```python
from build123d import *

# Parameters (mm, degrees)
SKETCH2_W                    = 600
SKETCH2_H                    = 812
BASE_FLANGE1_DEPTH           = 2
EDGE_FLANGE1_STRIP_W         = 9
EDGE_FLANGE1_STRIP_H         = 2
EDGE_FLANGE1_STRIP_CUT_DEPTH = 600
EDGE_FLANGE1_DEPTH           = 600
EDGE_FLANGE3_DEPTH           = 809.5
EDGE_FLANGE4_DEPTH           = 809.5
EDGE_FLANGE5_DEPTH           = 600
SKETCH22_R                   = 2.5
CUT_EXTRUDE1_DEPTH           = 870.278724001
SKETCH23_R                   = 2.5
CUT_EXTRUDE2_DEPTH           = 870.278724001
SKETCH24_R                   = 2.5
CUT_EXTRUDE3_DEPTH           = 25
EDGE_FLANGE6_STRIP_W         = 10
EDGE_FLANGE6_STRIP_H         = 2
EDGE_FLANGE6_STRIP_CUT_DEPTH = 809.5
EDGE_FLANGE6_DEPTH           = 809.5
EDGE_FLANGE7_STRIP_W         = 10
EDGE_FLANGE7_STRIP_H         = 2
EDGE_FLANGE7_STRIP_CUT_DEPTH = 809.5
EDGE_FLANGE7_DEPTH           = 809.5
EDGE_FLANGE8_STRIP_W         = 10
EDGE_FLANGE8_STRIP_H         = 2
EDGE_FLANGE8_STRIP_CUT_DEPTH = 809.5
EDGE_FLANGE8_DEPTH           = 809.5
EDGE_FLANGE9_STRIP_W         = 10
EDGE_FLANGE9_STRIP_H         = 2
EDGE_FLANGE9_STRIP_CUT_DEPTH = 809.5
EDGE_FLANGE9_DEPTH           = 809.5


# Sheet-metal steps are written as plain solids
with BuildPart() as part:
    # Sketch2 → Base-Flange1 (new body)
    with BuildSketch(Plane(origin=(0, 0, 0), x_dir=(0, 0, -1), z_dir=(1, 0, 0))):
        Rectangle(SKETCH2_W, SKETCH2_H)
    extrude(amount=-BASE_FLANGE1_DEPTH)

    # Edge-Flange1 strip (across the edge) → Edge-Flange1 strip cut (cut)
    with BuildSketch(Plane(origin=(-2, 406, 300), x_dir=(0, -1, 0), z_dir=(0, 0, -1))):
        with Locations((-2, -1)):
            Rectangle(EDGE_FLANGE1_STRIP_W, EDGE_FLANGE1_STRIP_H)
    extrude(amount=EDGE_FLANGE1_STRIP_CUT_DEPTH, mode=Mode.SUBTRACT)

    # Edge-Flange1 section (across the edge) → Edge-Flange1 (add)
    with BuildSketch(Plane(origin=(-2, 406, 300), x_dir=(0, -1, 0), z_dir=(0, 0, -1))):
        with BuildLine():
            Line((0, 0.5), (0, 25))
            Line((0, 25), (2, 25))
            Line((2, 25), (2, 0.5))
            ThreePointArc((2, 0.5), (2.146446609, 0.146446609), (2.5, 0))
            Line((2.5, 0), (2.5, -2))
            ThreePointArc((2.5, -2), (0.732233047, -1.267766953), (0, 0.5))
        make_face()
    extrude(amount=EDGE_FLANGE1_DEPTH)

    # Edge-Flange3 section (across the edge) → Edge-Flange3 (add)
    with BuildSketch(Plane(origin=(-2, -406, 300.5), x_dir=(0, 0, -1), z_dir=(0, 1, 0))):
        with BuildLine():
            Line((-2, 0.5), (-2, 25))
            Line((-2, 25), (0, 25))
            Line((0, 25), (0, 0.5))
            ThreePointArc((0, 0.5), (0.146446609, 0.146446609), (0.5, 0))
            Line((0.5, 0), (0.5, -2))
            ThreePointArc((0.5, -2), (-1.267766953, -1.267766953), (-2, 0.5))
        make_face()
    extrude(amount=EDGE_FLANGE3_DEPTH)

    # Edge-Flange4 section (across the edge) → Edge-Flange4 (add)
    with BuildSketch(Plane(origin=(-2, 403.5, -300.5), x_dir=(0, 0, 1), z_dir=(0, -1, 0))):
        with BuildLine():
            Line((-2, 0.5), (-2, 25))
            Line((-2, 25), (0, 25))
            Line((0, 25), (0, 0.5))
            ThreePointArc((0, 0.5), (0.146446609, 0.146446609), (0.5, 0))
            Line((0.5, 0), (0.5, -2))
            ThreePointArc((0.5, -2), (-1.267766953, -1.267766953), (-2, 0.5))
        make_face()
    extrude(amount=EDGE_FLANGE4_DEPTH)

    # Edge-Flange5 section (across the edge) → Edge-Flange5 (add)
    with BuildSketch(Plane(origin=(-2, -406.5, -300), x_dir=(0, 1, 0), z_dir=(0, 0, 1))):
        with BuildLine():
            Line((-2, 0.5), (-2, 25))
            Line((-2, 25), (0, 25))
            Line((0, 25), (0, 0.5))
            ThreePointArc((0, 0.5), (0.146446609, 0.146446609), (0.5, 0))
            Line((0.5, 0), (0.5, -2))
            ThreePointArc((0.5, -2), (-1.267766953, -1.267766953), (-2, 0.5))
        make_face()
    extrude(amount=EDGE_FLANGE5_DEPTH)

    # Sketch22 → Cut-Extrude1 (cut, through all)
    with BuildSketch(Plane.XZ.offset(408.5)):
        with Locations((-22, 278.5)):
            Circle(SKETCH22_R)
    extrude(amount=-CUT_EXTRUDE1_DEPTH, mode=Mode.SUBTRACT)

    # Sketch23 → Cut-Extrude2 (cut, through all)
    with BuildSketch(Plane(origin=(0, 406, 0), x_dir=(1, 0, 0), z_dir=(0, 1, 0))):
        with Locations(Location((-22, 278.5, 0), (0, 0, 180))):
            Circle(SKETCH23_R)
    extrude(amount=-CUT_EXTRUDE2_DEPTH, mode=Mode.SUBTRACT)

    # Sketch24 → Cut-Extrude3 (cut)
    with BuildSketch(Plane(origin=(0, 0, -302.5), x_dir=(-1, 0, 0), z_dir=(0, 0, -1))):
        with Locations((22, 382)):
            Circle(SKETCH24_R)
        with Locations((22, -384.5)):
            Circle(SKETCH24_R)
    extrude(amount=-CUT_EXTRUDE3_DEPTH, mode=Mode.SUBTRACT)

    # Edge-Flange6 strip (across the edge) → Edge-Flange6 strip cut (cut)
    with BuildSketch(Plane(origin=(-27, 403.5, -300.5), x_dir=(1, 0, 0), z_dir=(0, -1, 0))):
        with Locations((-4, -1)):
            Rectangle(EDGE_FLANGE6_STRIP_W, EDGE_FLANGE6_STRIP_H)
    extrude(amount=EDGE_FLANGE6_STRIP_CUT_DEPTH, mode=Mode.SUBTRACT)

    # Edge-Flange6 section (across the edge) → Edge-Flange6 (add)
    with BuildSketch(Plane(origin=(-27, 403.5, -300.5), x_dir=(1, 0, 0), z_dir=(0, -1, 0))):
        with BuildLine():
            Line((-2, 1), (-2, 10))
            Line((-2, 10), (0, 10))
            Line((0, 10), (0, 1))
            ThreePointArc((0, 1), (0.292893219, 0.292893219), (1, 0))
            Line((1, 0), (1, -2))
            ThreePointArc((1, -2), (-1.121320344, -1.121320344), (-2, 1))
        make_face()
    extrude(amount=EDGE_FLANGE6_DEPTH)

    # Edge-Flange7 strip (across the edge) → Edge-Flange7 strip cut (cut)
    with BuildSketch(Plane(origin=(-27, 403.5, -290.5), x_dir=(0, 0, -1), z_dir=(0, -1, 0))):
        with Locations((-4, -1)):
            Rectangle(EDGE_FLANGE7_STRIP_W, EDGE_FLANGE7_STRIP_H)
    extrude(amount=EDGE_FLANGE7_STRIP_CUT_DEPTH, mode=Mode.SUBTRACT)

    # Edge-Flange7 section (across the edge) → Edge-Flange7 (add)
    with BuildSketch(Plane(origin=(-27, 403.5, -290.5), x_dir=(0, 0, -1), z_dir=(0, -1, 0))):
        with BuildLine():
            Line((-2, 1), (-2, 20))
            Line((-2, 20), (0, 20))
            Line((0, 20), (0, 1))
            ThreePointArc((0, 1), (0.292893219, 0.292893219), (1, 0))
            Line((1, 0), (1, -2))
            ThreePointArc((1, -2), (-1.121320344, -1.121320344), (-2, 1))
        make_face()
    extrude(amount=EDGE_FLANGE7_DEPTH)

    # Edge-Flange8 strip (across the edge) → Edge-Flange8 strip cut (cut)
    with BuildSketch(Plane(origin=(-27, -406, 300.5), x_dir=(1, 0, 0), z_dir=(0, 1, 0))):
        with Locations((-4, -1)):
            Rectangle(EDGE_FLANGE8_STRIP_W, EDGE_FLANGE8_STRIP_H)
    extrude(amount=EDGE_FLANGE8_STRIP_CUT_DEPTH, mode=Mode.SUBTRACT)

    # Edge-Flange8 section (across the edge) → Edge-Flange8 (add)
    with BuildSketch(Plane(origin=(-27, -406, 300.5), x_dir=(1, 0, 0), z_dir=(0, 1, 0))):
        with BuildLine():
            Line((-2, 1), (-2, 10))
            Line((-2, 10), (0, 10))
            Line((0, 10), (0, 1))
            ThreePointArc((0, 1), (0.292893219, 0.292893219), (1, 0))
            Line((1, 0), (1, -2))
            ThreePointArc((1, -2), (-1.121320344, -1.121320344), (-2, 1))
        make_face()
    extrude(amount=EDGE_FLANGE8_DEPTH)

    # Edge-Flange9 strip (across the edge) → Edge-Flange9 strip cut (cut)
    with BuildSketch(Plane(origin=(-27, -406, 290.5), x_dir=(0, 0, 1), z_dir=(0, 1, 0))):
        with Locations((-4, -1)):
            Rectangle(EDGE_FLANGE9_STRIP_W, EDGE_FLANGE9_STRIP_H)
    extrude(amount=EDGE_FLANGE9_STRIP_CUT_DEPTH, mode=Mode.SUBTRACT)

    # Edge-Flange9 section (across the edge) → Edge-Flange9 (add)
    with BuildSketch(Plane(origin=(-27, -406, 290.5), x_dir=(0, 0, 1), z_dir=(0, 1, 0))):
        with BuildLine():
            Line((-2, 1), (-2, 20))
            Line((-2, 20), (0, 20))
            Line((0, 20), (0, 1))
            ThreePointArc((0, 1), (0.292893219, 0.292893219), (1, 0))
            Line((1, 0), (1, -2))
            ThreePointArc((1, -2), (-1.121320344, -1.121320344), (-2, 1))
        make_face()
    extrude(amount=EDGE_FLANGE9_DEPTH)


solid = part.part
```
Design review of the part built by this model. Coordinates are the model's own, in mm. A direction names the side the tool comes from. Coordinates: 2 decimals unless noted, no trailing zeros. Order: outer loops, then holes, each group sorted by start corner. A loop starts at its lowest first (then second) coordinate and runs counter-clockwise, first axis right, second up. Notation, with made-up numbers: (-6, 20) - (45, 20) arc R14 cw to (45, 33) - close; hole circle Ø4 at (38.25, -27.75). An arc over 180 degrees is marked (long way). One line per question, with ' | ' between items.
Q1. Consider section A-A, the plane z = -34. Give the boundary of the cut face in (x, y).
Answer key:
outline: (-27, -408.5) - (-2.5, -408.5) arc R2.5 ccw to (0, -406) - (0, 403.5) arc R2.5 ccw to (-2.5, 406) - (-27, 406) - (-27, 404) - (-2.5, 404) arc R0.5 cw to (-2, 403.5) - (-2, -406) arc R0.5 cw to (-2.5, -406.5) - (-27, -406.5) - close
Q2. Consider section B-B, the plane y = 38. Give the boundary of the cut face in (x, z), then the cut area to 3 significant figures.
Answer key:
outline: (-29, -299.5) arc R3 ccw to (-26, -302.5) - (-2.5, -302.5) arc R2.5 ccw to (0, -300) - (0, 300) arc R2.5 ccw to (-2.5, 302.5) - (-26, 302.5) arc R3 ccw to (-29, 299.5) - (-29, 291.5) arc R3 ccw to (-26, 288.5) - (-7, 288.5) - (-7, 290.5) - (-26, 290.5) arc R1 cw to (-27, 291.5) - (-27, 299.5) arc R1 cw to (-26, 300.5) - (-2.5, 300.5) arc R0.5 cw to (-2, 300) - (-2, -300) arc R0.5 cw to (-2.5, -300.5) - (-26, -300.5) arc R1 cw to (-27, -299.5) - (-27, -291.5) arc R1 cw to (-26, -290.5) - (-7, -290.5) - (-7, -288.5) - (-26, -288.5) arc R3 ccw to (-29, -291.5) - close | area: 1,440 mm2
Q3. Clearance check with flat-ended pins moving along their axes: pin 1 Ø10 at (y, z) = (-316.5, 147.5) entering from +X; pin 2 Ø1.6 at (y, z) = (-407.5, -144) entering from -X; pin 3 Ø3 at (y, z) = (-316.5, -40.5) entering from -X. State where each tip first meets the part, or that it passes through.
Answer key:
pin 1: stops at x = 0 | pin 2: stops at x = -27 | pin 3: stops at x = -2
Q4. For faces 5 (the flat face through (-17, 4, -288.5)), 6 (the flat face through (-16, -7, 290.5)), 7 (the flat face through (-15, 406, 4)), list the 3-axis set-ups (+Z, -Z, +X, -X, +Y, -Y) from which the entire face can be reached by the end or side of a thin tool; tool diameter is ignored.
Answer key:
face 5: -X | face 6: none | face 7: +Z, -Z, +X, -X, +Y
Q5. To check wall thickness, follow line 1 along Z through (x, y) = (-22, 405.65); line 2 along Z through (x, y) = (-8.25, 38.5); line 3 along Y through (x, z) = (-22, -301.2). State the ranges of each line that lie inside material, in increasing order.
Answer key:
line 1: z = -300 to -281, -276 to 276, 281 to 300 | line 2: z = -302.5 to -300.5, -290.5 to -288.5, 288.5 to 290.5, 300.5 to 302.5 | line 3: y = -406 to -387, -382 to 379.5, 384.5 to 403.5
Q6. The part is to be moulded in two halves that separate along Z. For faces 1 (the flat face through (-2, 4, 4)), 2 (the flat face through (-14, 4, -302.5)), 3 (the flat face through (-15, -408.5, -4)), 4 (the flat face through (-17, -7, 288.5)), say which applies: +Z half, -Z half, draft (parallel to the pull), parting line (faces both ways), or undercut.
Answer key:
face 1: undercut | face 2: -Z half | face 3: draft | face 4: undercut
